Source: CAD feature listing. Evaluate the final solid. Frame: model axes, mm. Round coordinates to 2 decimals unless told otherwise and drop trailing zeros. Write each loop counter-clockwise with the first axis right and the second up, starting at its lowest first coordinate (ties: lowest second). Pieces come first, ordered by that corner, then holes.
```python
from build123d import *

# Parameters (mm, degrees)
BOSS_EXTRUDE1_DEPTH = 3.175
FILLET1_R           = 3.175
CUT_EXTRUDE1_DEPTH  = 4.175
FILLET2_R           = 12.7
FILLET3_R           = 6.35


with BuildPart() as part:
    # Sketch1 → Boss-Extrude1 (new body)
    with BuildSketch(Plane(origin=(0, 0, 0), x_dir=(1, 0, 0), z_dir=(0, 1, 0))):
        with BuildLine():
            Line((-287.3375, -5.894090512), (-287.3375, -292.1))
            Line((-287.3375, -292.1), (287.3375, -292.1))
            Line((287.3375, -292.1), (287.3375, 203.2))
            Line((287.3375, 203.2), (261.9375, 203.2))
            Line((261.9375, 203.2), (261.9375, 0))
            ThreePointArc((261.9375, 0), (0, -261.9375), (-261.9375, 0))
            Line((-261.9375, 0), (-261.9375, 38.1))
            Line((-261.9375, 38.1), (-287.3375, -5.894090512))
        make_face()
    extrude(amount=BOSS_EXTRUDE1_DEPTH)

    # Fillet1
    fillet1_edges = [part.edges().sort_by_distance(p)[0] for p in [
        (-261.9375, 1.5875, -38.1),
    ]]
    fillet(fillet1_edges, radius=FILLET1_R)

    # Sketch2 → Cut-Extrude1 (cut, through all)
    with BuildSketch(Plane(origin=(0, 3.175, 0), x_dir=(1, 0, 0), z_dir=(0, 1, 0))):
        Polygon((287.3375, -292.1), (122.2375, -292.1), (287.3375, -127), align=None)
        Polygon((-287.3375, -292.1), (-122.2375, -292.1), (-287.3375, -127), align=None)
    extrude(amount=-CUT_EXTRUDE1_DEPTH, mode=Mode.SUBTRACT)

    # Fillet2
    fillet2_edges = [part.edges().sort_by_distance(p)[0] for p in [
        (-287.3375, 1.5875, 5.894090512),
        (287.3375, 1.5875, 127),
        (122.2375, 1.5875, 292.1),
        (-287.3375, 1.5875, 127),
        (-122.2375, 1.5875, 292.1),
    ]]
    fillet(fillet2_edges, radius=FILLET2_R)

    # Fillet3
    fillet3_edges = [part.edges().sort_by_distance(p)[0] for p in [
        (261.9375, 1.5875, -203.2),
        (287.3375, 1.5875, -203.2),
    ]]
    fillet(fillet3_edges, radius=FILLET3_R)


solid = part.part
```
Q1. Line query: line 1 (X direction, y = 1.6, z = -178); line 2 (X direction, y = 2.85, z = 164.5); line 3 (X direction, y = 2.55, z = 133). Output: solid intervals per line, ascending.
Q2. Mould query, pull axis X, two halves, no side actions, for faces 1 (the face through (-276.6, 1.6, -12.7)), 2 (the face through (5.76, 1.565, 261.874)), 3 (the face through (20, 3.175, 263)), 4 (the face through (203.684, 1.61, 210.654)). Classes: pulls with the +X half, pulls with the -X half, needs draft (parallel to the pull), parting line crosses it, or undercut.
Q3. Section query D-D, the plane z = -158.5. Output: boundary loops of the cut face in (x, y) (1 decimal), and give its area (3 significant figures).
Q4. Pin query (flat end, axial travel): P1, Ø1.5, axis at x = 31, y = 2.5, coming from the -Z side; P2, Ø1.6, axis at y = 1, z = -106, coming from the -X side. Return the tip coordinate at first contact, or that it passes through.
Q5. Section query C-C, the plane x = 0. Output: boundary loops of the cut face in (y, z) (1 decimal).
Q6. Section query A-A, the plane z = -16.5. Output: boundary loops of the cut face in (x, y) (1 decimal), and give its area (3 significant figures).
Filled in:
1. line 1: x = 261.94 to 287.34
1. line 2: x = -249.84 to -203.84, 203.84 to 249.84
1. line 3: x = -281.34 to -225.66, 225.66 to 281.34
2. face 1: pulls with the -X half
2. face 2: undercut
2. face 3: needs draft
2. face 4: pulls with the +X half
3. outline: (261.9, 0) - (287.3, 0) - (287.3, 3.2) - (261.9, 3.2) - close
3. area: 80.6 mm2
4. P1: stops at z = 260.01
4. P2: stops at x = 261.94
5. outline: (0, 261.9) - (3.2, 261.9) - (3.2, 292.1) - (0, 292.1) - close
6. outline: (-274.4, 0) - (-261.9, 0) - (-261.9, 3.2) - (-274.4, 3.2) - close; (261.9, 0) - (287.3, 0) - (287.3, 3.2) - (261.9, 3.2) - close
6. area: 120 mm2
